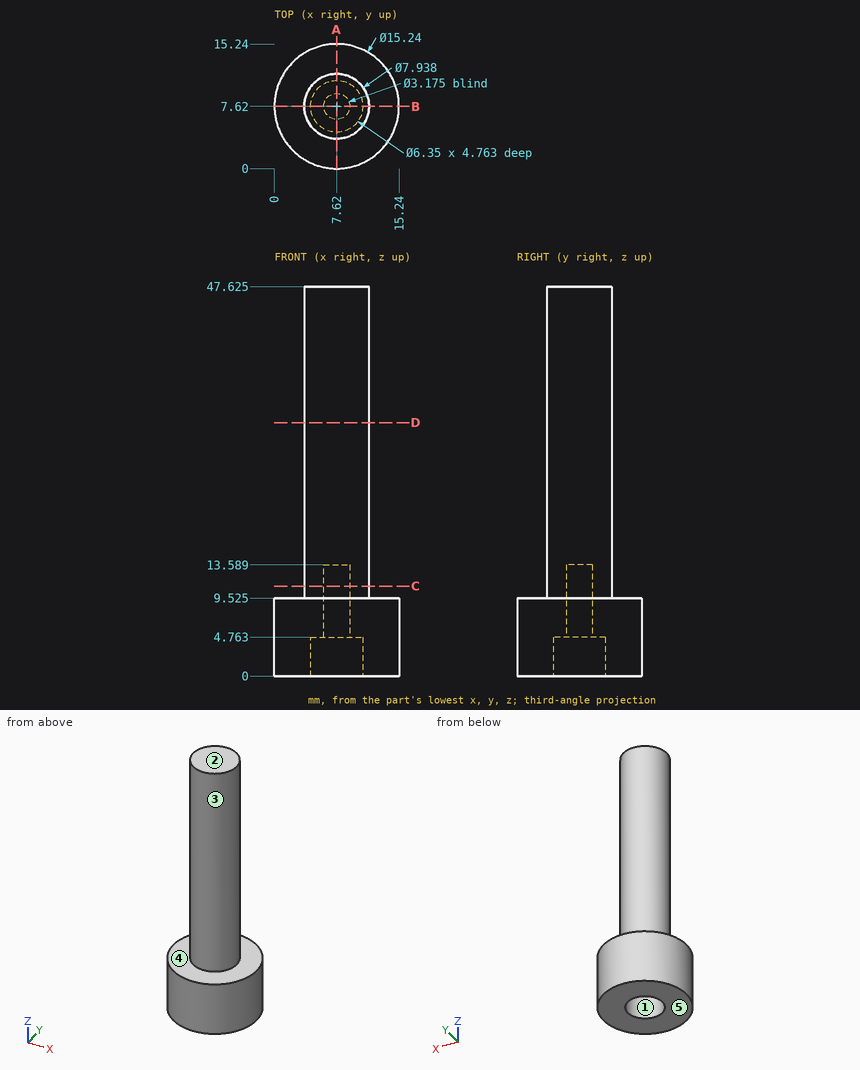
For this review, use the dimensioned drawing (mm, ordinates from the lowest corner) and the shaded views. A direction names the side the tool comes from. Round coordinates to 2 decimals unless told otherwise and drop trailing zeros. Order: outer loops, then holes, each group sorted by start corner. A loop starts at its lowest first (then second) coordinate and runs counter-clockwise, first axis right, second up. Notation, with made-up numbers: (67, 62) -> (100, 62) arc R23 ccw to (100, 91) -> close; hole circle Ø5 at (-18, -5.5). An arc over 180 degrees is marked (long way). Put each result on its own line as item: value.
Q1. For probe 1 along X at (y, z) = (7.75, 8); probe 2 along Y at (x, z) = (7.62, 3.5) (1 decimal); probe 3 along X at (y, z) = (7.75, 3.5), list the stretches that pass through material, from the lowest coordinate up. Write a range as [from, to].
Check result:
probe 1: [0, 6.04], [9.2, 15.24]
probe 2: [0, 4.4], [10.8, 15.2]
probe 3: [0, 4.45], [10.79, 15.24]
Q2. Add section A-A on x = 7.62. Write out the cut boundary in (y, z) (1 decimal).
Check result:
outline: (0, 0) -> (4.4, 0) -> (4.4, 4.8) -> (6, 4.8) -> (6, 13.6) -> (9.2, 13.6) -> (9.2, 4.8) -> (10.8, 4.8) -> (10.8, 0) -> (15.2, 0) -> (15.2, 9.5) -> (11.6, 9.5) -> (11.6, 47.6) -> (3.7, 47.6) -> (3.7, 9.5) -> (0, 9.5) -> close
Q3. Machinability: for the marked faces 4 and 5, which of the approach directions +Z, -Z, +X, -X, +Y, -Y give a long, thin tool a straight path to every point of the face, cutting with its end or side? Answer none if there is none.
Check result:
face 4: +Z
face 5: -Z, +X, -X, +Y, -Y
Q4. Mouldability with a two-part tool opening along X and no side actions: class the marked faces 1, 2 and 3 as pulls with the +X half, pulls with the -X half, needs draft (parallel to the pull), parting line crosses it, or undercut.
Check result:
face 1: undercut
face 2: needs draft
face 3: parting line crosses it
Q5. Add section D-D on z = 31. Write out the cut boundary in (x, y), plus the area to 3 significant figures.
Check result:
outline: circle Ø7.94 at (7.62, 7.62)
area: 49.5 mm2
Q6. Add section C-C on z = 11. Write out the cut boundary in (x, y) (1 decimal).
Check result:
outline: circle Ø7.9 at (7.6, 7.6); hole circle Ø3.2 at (7.6, 7.6)
Q7. Insertion check: pin 1 Ø3.5 at (x, y) = (8, 7) entering from -Z; pin 2 Ø4 at (y, z) = (4, 42) entering from +X; pin 3 Ø3 at (y, z) = (12, 27) entering from +X. Each pin has a flat end and moves straight along its axis. Give the tip position at first contact, or say it passes through.
Check result:
pin 1: z = 4.76
pin 2: x = 11.24
pin 3: x = 10.35
